CAD build for the part. Positions are in the model's coordinates, mm. Face numbers are marked on the shaded views. A direction names the side the tool comes from. Give positions to 0.01 mm unless a question says otherwise; leave off trailing zeros. Loops run counter-clockwise (first coordinate to the right, second up) from the corner with the lowest first, then second, coordinate; pieces in that order, holes last. Notation, with made-up numbers: M -17,35.5 L 38,35.5 A7 cw 38,45.5 Z; hole C 16.5,23.5 d2. An arc over 180 degrees is marked long. Answer as CSV lines item,"result".
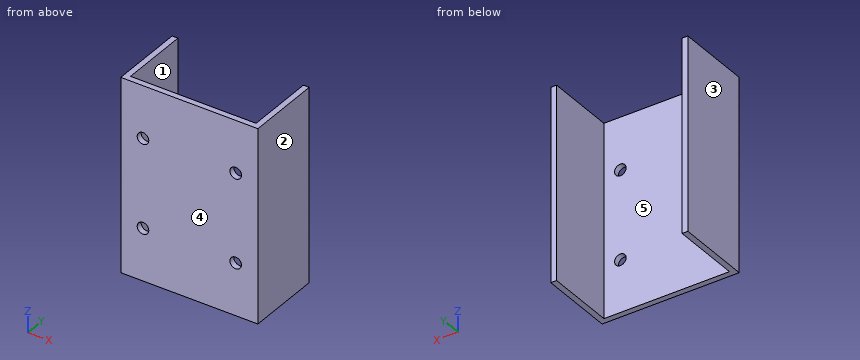
```python
from build123d import *

# Parameters (mm, degrees)
EXTRU_MINCE1_DEPTH      = 25
ESQUISSE2_R             = 1.5
ENL_V_MAT_EXTRU_1_DEPTH = 3


with BuildPart() as part:
    # Esquisse1 → Extru.-Mince1 (new, symmetric)
    with BuildSketch(Plane.XY):
        Polygon((-17.75, 19.5), (-17.75, 0), (17.75, 0), (17.75, 19.5), (16.25, 19.5), (16.25, 1.5), (-16.25, 1.5), (-16.25, 19.5), align=None)
    extrude(amount=EXTRU_MINCE1_DEPTH, both=True)

    # Esquisse2 → Enlèv. mat.-Extru.1 (cut)
    with BuildSketch(Plane.XZ):
        with Locations(Location((-12, 11.5, 0), (0, 0, 270))):
            Circle(ESQUISSE2_R)
        with Locations(Location((-12, -11.5, 0), (0, 0, 90))):
            Circle(ESQUISSE2_R)
        with Locations(Location((12, -11.5, 0), (0, 0, 270))):
            Circle(ESQUISSE2_R)
        with Locations(Location((12, 11.5, 0), (0, 0, 90))):
            Circle(ESQUISSE2_R)
    extrude(amount=-ENL_V_MAT_EXTRU_1_DEPTH, mode=Mode.SUBTRACT)


solid = part.part
```
Q1. Cut at C-C (x = 12). Write the cut outline in (y, z).
Solution:
outline,"M 0,-25 L 1.5,-25 L 1.5,-13 L 0,-13 Z; M 0,-10 L 1.5,-10 L 1.5,10 L 0,10 Z; M 0,13 L 1.5,13 L 1.5,25 L 0,25 Z"
Q2. Cut at A-A (z = -11.5). Write the cut outline in (x, y).
Solution:
outline,"M -17.75,0 L -13.5,0 L -13.5,1.5 L -16.25,1.5 L -16.25,19.5 L -17.75,19.5 Z; M -10.5,0 L 10.5,0 L 10.5,1.5 L -10.5,1.5 Z; M 13.5,0 L 17.75,0 L 17.75,19.5 L 16.25,19.5 L 16.25,1.5 L 13.5,1.5 Z"
Q3. Wall check: line 1 (X direction, y = 0.9, z = 11.5); line 2 (X direction, y = 15.75, z = 4.5); line 3 (Y direction, x = 2.5, z = -13.5). Give the ranges that are in metal, low to high. Write a range as [from, to].
Solution:
line 1,"x = [-17.75, -13.5], [-10.5, 10.5], [13.5, 17.75]"
line 2,"x = [-17.75, -16.25], [16.25, 17.75]"
line 3,"y = [0, 1.5]"
Q4. Which spindle directions (+Z, -Z, +X, -X, +Y, -Y) get a long thin tool onto all of the face, cutting with end or side? Do the marked faces 4 and 5. Say none if no direction does.
Solution:
face 4,"+Z, -Z, +X, -X, -Y"
face 5,"+Z, -Z, +Y"
Q5. Pin check, flat tips, straight feed: P1, Ø2.5, axis at x = -12, z = 11.5, coming from the +Y side; P2, Ø10, axis at x = -4.5, z = 4, coming from the +Y side. Stop position of each tip, or through.
Solution:
P1,"passes through"
P2,"stops at y = 1.5"
Q6. Cut at B-B (y = 4.5). Write the cut outline in (x, z), and give its area (3 significant figures).
Solution:
outline,"M -17.75,-25 L -16.25,-25 L -16.25,25 L -17.75,25 Z; M 16.25,-25 L 17.75,-25 L 17.75,25 L 16.25,25 Z"
area,"150 mm²"
Q7. Mould opens along X. For the marked faces 1, 2 and 3 say: released by +X, released by -X, zero draft, split by the parting line, or undercut.
Solution:
face 1,"undercut"
face 2,"released by +X"
face 3,"released by -X"
Q8. Cut at D-D (z = 20.5). Write the cut outline in (x, y), and give its area (3 significant figures).
Solution:
outline,"M -17.75,0 L 17.75,0 L 17.75,19.5 L 16.25,19.5 L 16.25,1.5 L -16.25,1.5 L -16.25,19.5 L -17.75,19.5 Z"
area,"107 mm²"
